Source: CAD feature listing. Evaluate the final solid. Frame: model axes, mm. A direction names the side the tool comes from. Round coordinates to 2 decimals unless told otherwise and drop trailing zeros. Loops run counter-clockwise (first coordinate to the right, second up) from the corner with the lowest first, then second, coordinate; pieces in that order, holes last. Notation, with made-up numbers: M -17.5,36 L 33.5,36 A22 cw 33.5,75 Z; hole C -25,59 d8. An arc over 180 degrees is marked long. One line per item, written item: value.
from build123d import *

# Parameters (mm, degrees)
SKETCH_6_R                         = 8
SKETCH_6_R_2                       = 1.65
SM_BASE_FLANGE_2_DEPTH             = 1.5
SM_EDGE_FLANGE_1_STRIP_W           = 7.4732
SM_EDGE_FLANGE_1_STRIP_H           = 1.5
SM_EDGE_FLANGE_1_STRIP_CUT_DEPTH   = 35
SM_EDGE_FLANGE_1_STRIP_2_W         = 7.4732
SM_EDGE_FLANGE_1_STRIP_2_H         = 1.5
SM_EDGE_FLANGE_1_STRIP_CUT_2_DEPTH = 35
SM_EDGE_FLANGE_1_DEPTH             = 35
SM_EDGE_FLANGE_1_BEND_DEPTH        = 35
CUT_EXTRUDE_1_DEPTH                = 76.828754441


# Sheet-metal steps are written as plain solids
with BuildPart() as part:
    # 草图6 → 基体-法兰2 (new body)
    with BuildSketch(Plane(origin=(0, 0, 0), x_dir=(1, 0, 0), z_dir=(0, 1, 0))):
        with BuildLine():
            Line((17.853571071, -17.5), (32.5, -17.5))
            Line((32.5, -17.5), (32.5, 17.5))
            Line((32.5, 17.5), (17.853571071, 17.5))
            ThreePointArc((17.853571071, 17.5), (0, 25), (-17.853571071, 17.5))
            Line((-17.853571071, 17.5), (-32.5, 17.5))
            Line((-32.5, 17.5), (-32.5, -17.5))
            Line((-32.5, -17.5), (-17.853571071, -17.5))
            ThreePointArc((-17.853571071, -17.5), (0, -25), (17.853571071, -17.5))
        make_face()
        with Locations(Location((0, 0, 0), (0, 0, 270))):
            Circle(SKETCH_6_R, mode=Mode.SUBTRACT)
        with Locations(Location((0, 15, 0), (0, 0, 270))):
            Circle(SKETCH_6_R_2, mode=Mode.SUBTRACT)
        with Locations(Location((-15, 0, 0), (0, 0, 270))):
            Circle(SKETCH_6_R_2, mode=Mode.SUBTRACT)
        with Locations(Location((0, -15, 0), (0, 0, 270))):
            Circle(SKETCH_6_R_2, mode=Mode.SUBTRACT)
        with Locations(Location((15, 0, 0), (0, 0, 270))):
            Circle(SKETCH_6_R_2, mode=Mode.SUBTRACT)
    extrude(amount=SM_BASE_FLANGE_2_DEPTH)

    # 边线-法兰1 strip (across the edge) → 边线-法兰1 strip cut (cut)
    with BuildSketch(Plane(origin=(-32.5, 1.5, -17.5), x_dir=(1, 0, 0), z_dir=(0, 0, 1))):
        with Locations((-1.5, -0.75)):
            Rectangle(SM_EDGE_FLANGE_1_STRIP_W, SM_EDGE_FLANGE_1_STRIP_H)
    extrude(amount=SM_EDGE_FLANGE_1_STRIP_CUT_DEPTH, mode=Mode.SUBTRACT)

    # 边线-法兰1 strip 2 (across the edge) → 边线-法兰1 strip cut 2 (cut)
    with BuildSketch(Plane(origin=(32.5, 1.5, 17.5), x_dir=(-1, 0, 0), z_dir=(0, 0, -1))):
        with Locations((-1.5, -0.75)):
            Rectangle(SM_EDGE_FLANGE_1_STRIP_2_W, SM_EDGE_FLANGE_1_STRIP_2_H)
    extrude(amount=SM_EDGE_FLANGE_1_STRIP_CUT_2_DEPTH, mode=Mode.SUBTRACT)

    # 边线-法兰1 section (across the edge) → 边线-法兰1 (add)
    with BuildSketch(Plane(origin=(-32.5, 1.5, -17.5), x_dir=(1, 0, 0), z_dir=(0, 0, 1))):
        with BuildLine():
            Line((0, 0.7366), (0, 28.5))
            Line((0, 28.5), (1.5, 28.5))
            Line((1.5, 28.5), (1.5, 0.7366))
            ThreePointArc((1.5, 0.7366), (1.715745145, 0.215745145), (2.2366, 0))
            Line((2.2366, 0), (2.2366, -1.5))
            ThreePointArc((2.2366, -1.5), (0.655084973, -0.844915027), (0, 0.7366))
        make_face()
    extrude(amount=SM_EDGE_FLANGE_1_DEPTH)

    # 边线-法兰1 section 2 (across the edge) → 边线-法兰1 bend (add)
    with BuildSketch(Plane(origin=(32.5, 1.5, 17.5), x_dir=(-1, 0, 0), z_dir=(0, 0, -1))):
        with BuildLine():
            Line((0, 0.7366), (0, 28.5))
            Line((0, 28.5), (1.5, 28.5))
            Line((1.5, 28.5), (1.5, 0.7366))
            ThreePointArc((1.5, 0.7366), (1.715745145, 0.215745145), (2.2366, 0))
            Line((2.2366, 0), (2.2366, -1.5))
            ThreePointArc((2.2366, -1.5), (0.655084973, -0.844915027), (0, 0.7366))
        make_face()
    extrude(amount=SM_EDGE_FLANGE_1_BEND_DEPTH)

    # 草图18 → 切除-拉伸1 (cut, through all)
    with BuildSketch(Plane(origin=(32.5, 0, 0), x_dir=(0, 0, -1), z_dir=(1, 0, 0))):
        with BuildLine():
            Line((-17.5, 30), (-17.5, 2.2366))
            Line((-17.5, 2.2366), (-4.434096645, 27.310581516))
            ThreePointArc((-4.434096645, 27.310581516), (-2.592980179, 29.275096933), (0, 30))
            Line((0, 30), (-17.5, 30))
        make_face()
        with BuildLine():
            Line((17.5, 30), (0, 30))
            ThreePointArc((0, 30), (2.592980179, 29.275096933), (4.434096645, 27.310581516))
            Line((4.434096645, 27.310581516), (17.5, 2.2366))
            Line((17.5, 2.2366), (17.5, 30))
        make_face()
        with BuildLine():
            ThreePointArc((2.15, 25), (1.52027958, 26.52027958), (0, 27.15))
            Line((0, 27.15), (0, 22.85))
            ThreePointArc((0, 22.85), (1.52027958, 23.47972042), (2.15, 25))
        make_face()
        with BuildLine():
            Line((0, 22.85), (0, 27.15))
            ThreePointArc((0, 27.15), (-2.15, 25), (0, 22.85))
        make_face()
        with BuildLine():
            ThreePointArc((2.15, 10), (1.52027958, 11.52027958), (0, 12.15))
            Line((0, 12.15), (0, 7.85))
            ThreePointArc((0, 7.85), (1.52027958, 8.47972042), (2.15, 10))
        make_face()
        with BuildLine():
            Line((0, 7.85), (0, 12.15))
            ThreePointArc((0, 12.15), (-2.15, 10), (0, 7.85))
        make_face()
    extrude(amount=-CUT_EXTRUDE_1_DEPTH, mode=Mode.SUBTRACT)


solid = part.part
1. Reachability of faces 4 (the face through (-25, 1, 17.5)), 5 (the face through (-13.364, 0.74, -0.215)), 6 (the face through (31, 13, 0)), 7 (the face through (-25, 1, -17.5)), 8 (the face through (25, 1, 17.5)) from +Z, -Z, +X, -X, +Y, -Y: full face, straight path, thin tool, end or side. Return the list, or none.
Report:
face 4: +Z, -X, +Y, -Y
face 5: +Y, -Y
face 6: +Z, -Z, +Y
face 7: -Z, -X, +Y, -Y
face 8: +Z, +X, +Y, -Y
2. Pin query (flat end, axial travel): pin 1 (1.8 mm diameter, centred on x = 26.5, y = 1, fed in from +Z); pin 2 (0.7 mm diameter, centred on x = -27, y = 1.5, fed in from -Z); pin 3 (4 mm diameter, centred on x = -7, z = -8, fed in from +Y). Return the tip coordinate at first contact, or that it passes through.
Report:
pin 1: stops at z = 17.5
pin 2: stops at z = -17.5
pin 3: stops at y = 1.5
3. Section query C-C (x = 15). Return the cut outline in (y, z).
Report:
outline: M 0,-20 L 1.5,-20 L 1.5,-1.65 L 0,-1.65 Z; M 0,1.65 L 1.5,1.65 L 1.5,20 L 0,20 Z
4. Section query D-D (z = 15). Return the cut outline in (x, y).
Report:
outline: M -32.5,2.24 A2.24 ccw -30.26,0 L -1.65,0 L -1.65,1.5 L -30.26,1.5 A0.74 cw -31,2.24 L -31,7.03 L -32.5,7.03 Z; M 1.65,0 L 30.26,0 A2.24 ccw 32.5,2.24 L 32.5,7.03 L 31,7.03 L 31,2.24 A0.74 cw 30.26,1.5 L 1.65,1.5 Z
5. Section query B-B (y = 11.25). Return the cut outline in (x, z), and give its area (3 significant figures).
Report:
outline: M -32.5,-12.8 L -31,-12.8 L -31,-1.75 L -32.5,-1.75 Z; M -32.5,1.75 L -31,1.75 L -31,12.8 L -32.5,12.8 Z; M 31,-12.8 L 32.5,-12.8 L 32.5,-1.75 L 31,-1.75 Z; M 31,1.75 L 32.5,1.75 L 32.5,12.8 L 31,12.8 Z
area: 66.3 mm2
6. Section query A-A (x = 0). Return the cut outline in (y, z).
Report:
outline: M 0,-25 L 1.5,-25 L 1.5,-16.65 L 0,-16.65 Z; M 0,-13.35 L 1.5,-13.35 L 1.5,-8 L 0,-8 Z; M 0,8 L 1.5,8 L 1.5,13.35 L 0,13.35 Z; M 0,16.65 L 1.5,16.65 L 1.5,25 L 0,25 Z
7. Ray query, line 1 (X direction, y = 5, z = -14.5); line 2 (X direction, y = 1.1, z = 0); line 3 (Y direction, x = 18.5, z = -1.5). Return the intervals inside material, ascending. Write a range as [from, to].
Report:
line 1: x = [-32.5, -31], [31, 32.5]
line 2: x = [-32.19, -16.65], [-13.35, -8], [8, 13.35], [16.65, 32.19]
line 3: y = [0, 1.5]
8. Pull-direction query (X, two-part tool) for faces 1 (the face through (-31.74, 14.598, 11.059)), 2 (the face through (0, 1, -25)), 3 (the face through (6, 1.5, -6)); classes: released by +X, released by -X, zero draft, split by the parting line, or undercut.
Report:
face 1: zero draft
face 2: split by the parting line
face 3: undercut
